```python
from build123d import *

# Parameters (mm, degrees)
F0_R     = 4.7625
F1_DEPTH = 41.91
F2_R     = 3.96875
F3_DEPTH = 38.1
F4_R     = 3.96875
F5_DEPTH = 1.27


with BuildPart() as f1:
    # F0 (on Front) → F1 (new body)
    with BuildSketch(Plane.XZ):
        Circle(F0_R)
    extrude(amount=F1_DEPTH)

    # F2 (on face) → F3 (cut)
    with BuildSketch(Plane(origin=(0, 0, 0), x_dir=(-1, 0, 0), z_dir=(0, 1, 0))):
        Circle(F2_R)
    extrude(amount=-F3_DEPTH, mode=Mode.SUBTRACT)

    # F4 (on face) → F5 (cut)
    with BuildSketch(Plane.XZ.offset(41.91)):
        Circle(F4_R)
    extrude(amount=-F5_DEPTH, mode=Mode.SUBTRACT)


solid = f1.part
```
Work out the finished part from the listing and answer in its coordinate system (mm). A direction names the side the tool comes from. Give positions to 0.01 mm unless a question says otherwise; leave off trailing zeros. Order: outer loops, then holes, each group sorted by start corner. A loop starts at its lowest first (then second) coordinate and runs counter-clockwise, first axis right, second up.
1. Section A-A, the plane z = 0 is taken. Determine the outline of the cut face in (x, y), and give its area (3 significant figures).
Result sheet:
outline: (-4.76, -41.91) - (-3.97, -41.91) - (-3.97, -40.64) - (3.97, -40.64) - (3.97, -41.91) - (4.76, -41.91) - (4.76, 0) - (3.97, 0) - (3.97, -38.1) - (-3.97, -38.1) - (-3.97, 0) - (-4.76, 0) - close
area: 86.7 mm2
2. The mould has two halves that part along X. Classify faces 1 (the cylindrical face through (-3.78, -20.66, -2.9)), 2 (the cylindrical face through (0.86, -18.783, -3.874)), 3 (the flat face through (-2, -41.91, 4)), 4 (the cylindrical face through (-0.86, -41.284, -3.874)): released by +X, released by -X, zero draft, split by the parting line, or undercut.
Result sheet:
face 1: split by the parting line
face 2: undercut
face 3: zero draft
face 4: undercut
3. Section C-C, the plane y = -20 is taken. Determine the outline of the cut face in (x, z) (1 decimal), and give its area (3 significant figures).
Result sheet:
outline: circle Ø9.5 at (0, 0); hole circle Ø7.9 at (0, 0)
area: 21.8 mm2
4. For faces 5 (the flat face through (0, -38.1, 0)), 6 (the flat face through (-2, 0, 4)), 7 (the flat face through (0, -40.64, 0)), determine the directions among +Z, -Z, +X, -X, +Y, -Y from which every point of the face is accessible in a straight line to the end or side of a thin tool.
Result sheet:
face 5: +Y
face 6: +Z, -Z, +X, -X, +Y
face 7: -Y
5. Straight lines are drawn through the part: L1, parallel to Z at x = 0, y = -26; L2, parallel to Y at x = -3, z = -2.5; L3, parallel to X at y = -11.5, z = 1. For each, find the intervals that lie inside material, in ascending order.
Result sheet:
L1: z = -4.76 to -3.97, 3.97 to 4.76
L2: y = -40.64 to -38.1
L3: x = -4.66 to -3.84, 3.84 to 4.66
6. Each of these flat-tipped pins is pushed along its axis until it touches: P1, Ø1, axis at y = -23.5, z = -1.5, coming from the -X side; P2, Ø2.5, axis at x = 0, z = 0.5, coming from the +Y side; P3, Ø2.5, axis at x = -0.5, z = 0, coming from the -Y side. Where does it stop, or does it pass through?
Result sheet:
P1: stops at x = -4.66
P2: stops at y = -38.1
P3: stops at y = -40.64
7. Section B-B, the plane x = 0 is taken. Determine the outline of the cut face in (y, z), and give its area (3 significant figures).
Result sheet:
outline: (-41.91, -4.76) - (0, -4.76) - (0, -3.97) - (-38.1, -3.97) - (-38.1, 3.97) - (0, 3.97) - (0, 4.76) - (-41.91, 4.76) - (-41.91, 3.97) - (-40.64, 3.97) - (-40.64, -3.97) - (-41.91, -3.97) - close
area: 86.7 mm2
